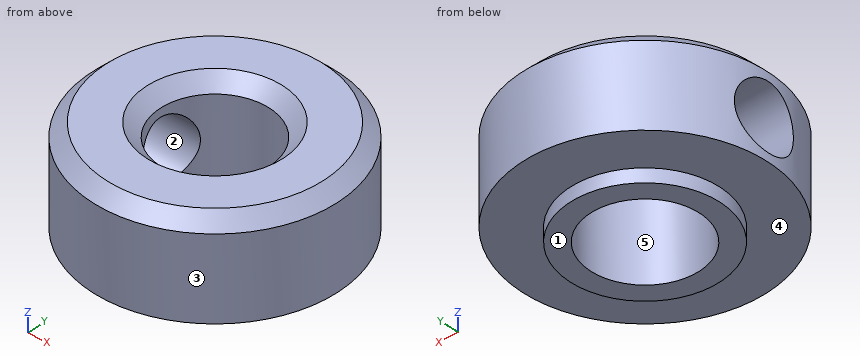
from build123d import *

# Parameters (mm, degrees)
CROQUIS1_R              = 9
SALIENTE_EXTRUIR1_DEPTH = 8
CROQUIS2_R              = 4
CORTAR_EXTRUIR1_DEPTH   = 16.033296378
CHAFL_N1_SIZE           = 1
CROQUIS3_R              = 2.38125
CORTAR_EXTRUIR2_DEPTH   = 10
CROQUIS4_R              = 11.390520889
CROQUIS4_R_2            = 5.5
CORTAR_EXTRUIR3_DEPTH   = 1


with BuildPart() as part:
    # Croquis1 → Saliente-Extruir1 (new body)
    with BuildSketch(Plane.XY):
        Circle(CROQUIS1_R)
    extrude(amount=SALIENTE_EXTRUIR1_DEPTH)

    # Croquis2 → Cortar-Extruir1 (cut, through all)
    with BuildSketch(Plane.XY.offset(8)):
        Circle(CROQUIS2_R)
    extrude(amount=-CORTAR_EXTRUIR1_DEPTH, mode=Mode.SUBTRACT)

    # Chaflán1
    chafl_n1_edges = [part.edges().sort_by_distance(p)[0] for p in [
        (-9, 0, 8),
        (-4, 0, 8),
    ]]
    chamfer(chafl_n1_edges, length=CHAFL_N1_SIZE)

    # Croquis3 → Cortar-Extruir2 (cut)
    with BuildSketch(Plane(origin=(0, 0, 0), x_dir=(0, 0, -1), z_dir=(1, 0, 0))):
        with Locations((-4, 0)):
            Circle(CROQUIS3_R)
    extrude(amount=-CORTAR_EXTRUIR2_DEPTH, mode=Mode.SUBTRACT)

    # Croquis4 → Cortar-Extruir3 (cut)
    with BuildSketch(Plane(origin=(0, 0, 0), x_dir=(-1, 0, 0), z_dir=(0, 0, -1))):
        Circle(CROQUIS4_R)
        Circle(CROQUIS4_R_2, mode=Mode.SUBTRACT)
    extrude(amount=-CORTAR_EXTRUIR3_DEPTH, mode=Mode.SUBTRACT)


solid = part.part
Input: part model. Units: mm. Frame: model coordinates. Face numbers are marked on the shaded views. A direction names the side the tool comes from. Round coordinates to 2 decimals unless told otherwise and drop trailing zeros. Write each loop counter-clockwise with the first axis right and the second up, starting at its lowest first coordinate (ties: lowest second). Pieces come first, ordered by that corner, then holes.
1) Ray query, L1, parallel to Y at x = 0, z = 4.5; L2, parallel to X at y = 0, z = 4.5; L3, parallel to X at y = -1.75, z = 2.25. Return the intervals inside material, ascending.
2) Reachability of the marked faces 4 and 5 from +Z, -Z, +X, -X, +Y, -Y: full face, straight path, thin tool, end or side. Return the list, or none.
3) Cut plane C-C (z = 3). Return the cut outline in (x, y).
4) Cut plane A-A (x = 0). Return the cut outline in (y, z), then the cut area to 3 significant figures.
5) Contact query for flat-ended pins moving along their axis: P1, Ø1.5, axis at x = -5.5, z = 4.5, coming from the -Y side; P2, Ø1, axis at x = 5, y = -5.5, coming from the -Z side; P3, Ø2, axis at y = -6, z = 4.5, coming from the -X side. Output: stop coordinate, or through.
6) Draft query along Y for the marked faces 1, 2 and 3. Return one class per face: pulls with the +Y half, pulls with the -Y half, needs draft (parallel to the pull), parting line crosses it, or undercut.
7) Cut plane D-D (z = 4). Return the cut outline in (x, y), then the cut area to 3 significant figures.
8) Cut plane B-B (y = 0). Return the cut outline in (x, z).
Geometry says:
1. L1: y = -9 to -4, 4 to 9
1. L2: x = 4 to 9
1. L3: x = -8.83 to -3.6, 3.6 to 8.83
2. face 4: -Z
2. face 5: +Z, -Z
3. outline: (-8.74, -2.16) arc R9 ccw (long way) to (-8.74, 2.16) - (-3.37, 2.16) arc R4 cw (long way) to (-3.37, -2.16) - close
4. outline: (-9, 1) - (-5.5, 1) - (-5.5, 0) - (-4, 0) - (-4, 7) - (-5, 8) - (-8, 8) - (-9, 7) - close; (4, 0) - (5.5, 0) - (5.5, 1) - (9, 1) - (9, 7) - (8, 8) - (5, 8) - (4, 7) - close
4. area: 71.0 mm2
5. P1: stops at y = -7.64
5. P2: stops at z = 1
5. P3: stops at x = -7.48
6. face 1: needs draft
6. face 2: undercut
6. face 3: parting line crosses it
7. outline: (-8.68, -2.38) arc R9 ccw (long way) to (-8.68, 2.38) - (-3.21, 2.38) arc R4 cw (long way) to (-3.21, -2.38) - close
7. area: 180 mm2
8. outline: (-9, 1) - (-5.5, 1) - (-5.5, 0) - (-4, 0) - (-4, 1.62) - (-9, 1.62) - close; (-9, 6.38) - (-4, 6.38) - (-4, 7) - (-5, 8) - (-8, 8) - (-9, 7) - close; (4, 0) - (5.5, 0) - (5.5, 1) - (9, 1) - (9, 7) - (8, 8) - (5, 8) - (4, 7) - close
